```python
from build123d import *

# Parameters (mm, degrees)
SKETCH1_R           = 62
BOSS_EXTRUDE1_DEPTH = 10
SKETCH2_R           = 6
CUT_EXTRUDE1_DEPTH  = 10
SKETCH4_W           = 44
SKETCH4_H           = 25
BOSS_EXTRUDE2_DEPTH = 25
BOSS_EXTRUDE5_DEPTH = 25
BOSS_EXTRUDE6_START = -25
BOSS_EXTRUDE6_DEPTH = 25
SKETCH9_R           = 15
CUT_EXTRUDE2_DEPTH  = 25
CUT_EXTRUDE3_START  = -25
SKETCH10_R          = 15
CUT_EXTRUDE3_DEPTH  = 25


with BuildPart() as part:
    # Sketch1 → Boss-Extrude1 (new body)
    with BuildSketch(Plane.XY):
        Circle(SKETCH1_R)
    extrude(amount=BOSS_EXTRUDE1_DEPTH)

    # Sketch2 → Cut-Extrude1 (cut)
    with BuildSketch(Plane.XY.offset(10)):
        with Locations((35.355339059, -35.355339059)):
            Circle(SKETCH2_R)
        with Locations((-35.355339059, -35.355339059)):
            Circle(SKETCH2_R)
        with Locations((-35.355339059, 35.355339059)):
            Circle(SKETCH2_R)
        with Locations((35.548908594, 35.160703886)):
            Circle(SKETCH2_R)
    extrude(amount=-CUT_EXTRUDE1_DEPTH, mode=Mode.SUBTRACT)

    # Sketch4 → Boss-Extrude2 (add)
    with BuildSketch(Plane.XY.offset(10)):
        with Locations((0, 43.5)):
            Rectangle(SKETCH4_W, SKETCH4_H)
        with Locations((0, -43.5)):
            Rectangle(SKETCH4_W, SKETCH4_H)
    extrude(amount=BOSS_EXTRUDE2_DEPTH)

    # Sketch5 → Boss-Extrude5 (add)
    with BuildSketch(Plane(origin=(0, 56, 0), x_dir=(1, 0, 0), z_dir=(0, 1, 0))):
        with BuildLine():
            Line((-22, -35), (22, -35))
            ThreePointArc((22, -35), (0, -57), (-22, -35))
        make_face()
    extrude(amount=-BOSS_EXTRUDE5_DEPTH)

    # Sketch8 → Boss-Extrude6 (add)
    with BuildSketch(Plane.XZ.offset(56).offset(BOSS_EXTRUDE6_START)):
        with BuildLine():
            Line((-22, 35), (22, 35))
            ThreePointArc((22, 35), (0, 57), (-22, 35))
        make_face()
    extrude(amount=BOSS_EXTRUDE6_DEPTH)

    # Sketch9 → Cut-Extrude2 (cut)
    with BuildSketch(Plane(origin=(0, 56, 0), x_dir=(1, 0, 0), z_dir=(0, 1, 0))):
        with Locations(Location((0, -35, 0), (0, 0, 270))):
            Circle(SKETCH9_R)
    extrude(amount=-CUT_EXTRUDE2_DEPTH, mode=Mode.SUBTRACT)

    # Sketch10 → Cut-Extrude3 (cut)
    with BuildSketch(Plane.XZ.offset(56).offset(CUT_EXTRUDE3_START)):
        with Locations(Location((0, 35, 0), (0, 0, 90))):
            Circle(SKETCH10_R)
    extrude(amount=CUT_EXTRUDE3_DEPTH, mode=Mode.SUBTRACT)


solid = part.part
```
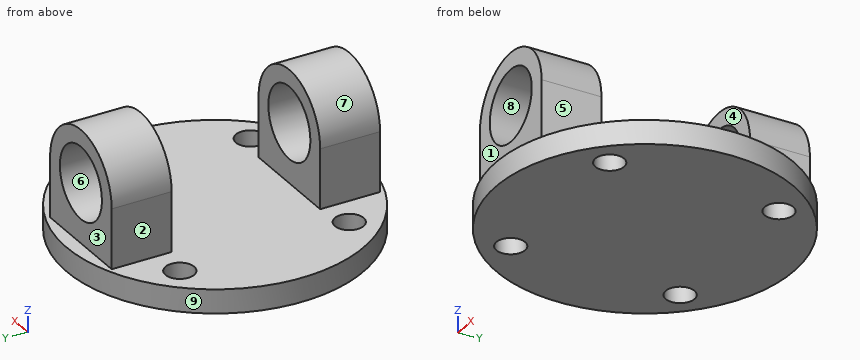
Input: part model. Units: mm. Frame: model coordinates. Face numbers are marked on the shaded views. A direction names the side the tool comes from. Give positions to 0.01 mm unless a question says otherwise; leave off trailing zeros. Order: outer loops, then holes, each group sorted by start corner. A loop starts at its lowest first (then second) coordinate and runs counter-clockwise, first axis right, second up.
1. Cut plane C-C (z = 21.5). Return loops of the section in (x, y), and give its area (3 significant figures).
Computed:
outline: (-22, -56) - (-6.54, -56) - (-6.54, -31) - (-22, -31) - close; (-22, 31) - (-6.54, 31) - (-6.54, 56) - (-22, 56) - close; (6.54, -56) - (22, -56) - (22, -31) - (6.54, -31) - close; (6.54, 31) - (22, 31) - (22, 56) - (6.54, 56) - close
area: 1,550 mm2
2. Line query: probe 1 along X at (y, z) = (37.75, 35); probe 2 along Y at (x, z) = (-18.5, 31); probe 3 along Y at (x, z) = (-38, 7.5). Output: solid intervals per line, ascending.
Computed:
probe 1: x = -22 to -15, 15 to 22
probe 2: y = -56 to -31, 31 to 56
probe 3: y = -48.99 to -40.74, -29.97 to 29.97, 40.74 to 48.99
3. Pin query (flat end, axial travel): pin 1 Ø13 at (x, z) = (-3, 27.5) entering from +Y; pin 2 Ø20 at (y, z) = (44, 24.5) entering from +X; pin 3 Ø8 at (x, y) = (37.5, 13.5) entering from +Z; pin 4 Ø12.5 at (y, z) = (-46.5, 17.5) entering from -X. Return the tip coordinate at first contact, or that it passes through.
Computed:
pin 1: passes through
pin 2: stops at x = 22
pin 3: stops at z = 10
pin 4: stops at x = -22
4. Cut plane D-D (y = 48.5). Return loops of the section in (x, z), and give its area (3 significant figures).
Computed:
outline: (-38.62, 0) - (38.62, 0) - (38.62, 10) - (22, 10) - (22, 35) arc R22 ccw to (-22, 35) - (-22, 10) - (-38.62, 10) - close; hole circle Ø30 at (0, 35)
area: 1,930 mm2
5. Draft query along Z for the marked faces 6, 7, 8 and 9. Return one class per face: released by +Z, released by -Z, zero draft, split by the parting line, or undercut.
Computed:
face 6: undercut
face 7: released by +Z
face 8: undercut
face 9: zero draft
6. Cut plane B-B (x = 0). Return loops of the section in (y, z), and give its area (3 significant figures).
Computed:
outline: (-62, 0) - (62, 0) - (62, 10) - (56, 10) - (56, 20) - (31, 20) - (31, 10) - (-31, 10) - (-31, 20) - (-56, 20) - (-56, 10) - (-62, 10) - close; (-56, 50) - (-31, 50) - (-31, 57) - (-56, 57) - close; (31, 50) - (56, 50) - (56, 57) - (31, 57) - close
area: 2,090 mm2
7. Cut plane A-A (z = 14). Return loops of the section in (x, y), and give its area (3 significant figures).
Computed:
outline: (-22, -56) - (22, -56) - (22, -31) - (-22, -31) - close; (-22, 31) - (22, 31) - (22, 56) - (-22, 56) - close
area: 2,200 mm2
8. Set-up query: the marked faces 1, 2, 3, 4 and 5. Return all of +Z, -Z, +X, -X, +Y, -Y with unobstructed straight access to the full face (end or side cutting, diameter ignored); none if empty.
Computed:
face 1: +Z, +X, -X, -Y
face 2: +Z, -X, +Y, -Y
face 3: +Z, +X, -X, +Y
face 4: +Z, +X, -X
face 5: +Z, +X, +Y, -Y
